Work out the finished part from the listing and answer in its coordinate system (mm). A direction names the side the tool comes from. Give positions to 0.01 mm unless a question says otherwise; leave off trailing zeros. Write each loop counter-clockwise with the first axis right and the second up, starting at its lowest first coordinate (ties: lowest second). Pieces come first, ordered by that corner, then holes. Notation, with made-up numbers: (-2.5, 41) -> (51.5, 41) arc R23 cw to (51.5, 60) -> close; hole circle Ø2 at (7, -38). An arc over 180 degrees is marked (long way). Use a Markdown table: item, result. Add a question column.
Q1. For a pull along Z with two mould halves and no side action, classify faces 1 (the face through (-6.2, -9.3, 0)), 2 (the face through (14, 0, 56)), 3 (the face through (-14, -8, 87)), 4 (the face through (13.57, -11.02, 38.6)) as pulls with the +Z half, pulls with the -Z half, needs draft (parallel to the pull), parting line crosses it, or undercut.
Q2. For faces 5 (the face through (18, -11, 25)), 6 (the face through (-12.27, -3.944, 27.444)), 7 (the face through (22.4, -6.41, 49.07)), 8 (the face through (-18, -7, 55)), determine the directions among +Z, -Z, +X, -X, +Y, -Y from which every point of the face is accessible in a straight line to the end or side of a thin tool.
Q3. Section B-B, the plane z = 56 is taken. Give the vertices of the cut face in (x, y) (3 decimals).
Q4. Each of these flat-tipped pins is pushed along its axis until it touches: pin 1 Ø6 at (x, z) = (-3.5, 17.5) entering from +Y; pin 2 Ø1.2 at (x, y) = (19, -11.5) entering from +Z; pin 3 Ø1.2 at (x, y) = (17.5, -11) entering from -Z; pin 4 Ø4.5 at (x, z) = (18, 31.5) entering from -Y. Where does it stop, or does it pass through?
Q5. Section C-C, the plane x = -14.5 is taken. Give the vertices of the cut face in (y, z) (3 decimals), plus the area to 3 significant figures.
Q6. Section D-D, the plane x = 0 is taken. Give the vertices of the cut face in (y, z), plus the area to 3 significant figures.
Q7. Section A-A, the plane z = 31.5 is taken. Give the vertices of the cut face in (x, y).
Q8. Consider line 1 (Z direction, x = 20.5, y = -9.25); line 2 (Z direction, x = -14.5, y = -2.5) (3 decimals); line 3 (Z direction, x = 18, y = -10.7). Determine where each line is inside the solid, lowest interval first.
from build123d import *

# Parameters (mm, degrees)
BOSS_EXTRUDE1_DEPTH  = 112
SKETCH2_R            = 3.025
CUT_EXTRUDE1_DEPTH   = 8
SKETCH3_W            = 11
SKETCH3_H            = 11
BOSS_EXTRUDE2_DEPTH  = 4
BOSS_EXTRUDE3_REACH  = 126.988
SKETCH8_W            = 10
SKETCH8_H            = 13
BOSS_EXTRUDE4_DEPTH  = 4
FILLET1_R            = 2
M4_CLEARANCE_HOLE1_D = 4.8
MIRROR1_START        = 12.831076745
MIRROR1_OUTLINE_W    = 4
MIRROR1_OUTLINE_H    = 13
MIRROR1_DEPTH        = 2.768923155
MIRROR1_START_2      = 20.4000001
MIRROR1_2_OUTLINE_W  = 4
MIRROR1_2_OUTLINE_H  = 13
MIRROR1_2_DEPTH      = 0.5999999
MIRROR1_START_3      = 74
MIRROR1_3_DEPTH      = 13
MIRROR1_4_OUTLINE_W  = 4.8000002
MIRROR1_4_OUTLINE_H  = 4
MIRROR1_4_DEPTH      = 4.0999999
MIRROR1_START_4      = 82.9000001
MIRROR1_5_OUTLINE_W  = 4.8000002
MIRROR1_5_OUTLINE_H  = 4
MIRROR1_5_DEPTH      = 4.0999999
MIRROR1_START_5      = 76
MIRROR1_6_OUTLINE_W  = 2
MIRROR1_6_OUTLINE_H  = 4
MIRROR1_6_DEPTH      = 9
MIRROR1_START_6      = -13
MIRROR1_7_DEPTH      = 4
CUT_EXTRUDE2_DEPTH   = 126.455171276
BOSS_EXTRUDE5_START  = -87
BOSS_EXTRUDE5_DEPTH  = 112
SKETCH15_W           = 10
SKETCH15_H           = 15
SKETCH15_R           = 3.025
BOSS_EXTRUDE6_DEPTH  = 13
SKETCH16_R           = 3.025
CUT_EXTRUDE3_DEPTH   = 8
FILLET2_R            = 2
FILLET3_R            = 1


with BuildPart() as part:
    # Sketch1 → Boss-Extrude1 (new body)
    with BuildSketch(Plane.XY):
        with BuildLine():
            ThreePointArc((0, -13), (-9.192388155, -9.192388155), (-13, 0))
            Line((-13, 0), (-18, 0))
            Line((-18, 0), (-18, -13))
            Line((-18, -13), (0, -13))
        make_face()
        with BuildLine():
            Line((-11, 0), (-13, 0))
            ThreePointArc((-13, 0), (-9.192388155, -9.192388155), (0, -13))
            ThreePointArc((0, -13), (9.192388155, -9.192388155), (13, 0))
            Line((13, 0), (11, 0))
            ThreePointArc((11, 0), (0, -11), (-11, 0))
        make_face()
    extrude(amount=BOSS_EXTRUDE1_DEPTH)

    # Sketch2 → Cut-Extrude1 (cut)
    with BuildSketch(Plane(origin=(0, 0, 0), x_dir=(1, 0, 0), z_dir=(0, 1, 0))):
        with Locations(Location((-14.5, -25.4, 0), (0, 0, 180))):
            Circle(SKETCH2_R)
        with Locations(Location((-14.5, -86.6, 0), (0, 0, 180))):
            Circle(SKETCH2_R)
    extrude(amount=-CUT_EXTRUDE1_DEPTH, mode=Mode.SUBTRACT)

    # Sketch3 → Boss-Extrude2 (add)
    with BuildSketch(Plane.XZ.offset(13)):
        with Locations((-12.5, 117.5)):
            Rectangle(SKETCH3_W, SKETCH3_H)
    extrude(amount=-BOSS_EXTRUDE2_DEPTH)

    # Sketch7 → Boss-Extrude3 (add, up to next)
    with BuildSketch(Plane.XZ.offset(13), mode=Mode.PRIVATE) as boss_extrude3_sk1:
        Polygon((0, 25), (13, 25), (13, 31.5), (13, 38), (0, 38), align=None)
    boss_extrude3_tool1 = extrude(boss_extrude3_sk1.sketch, amount=-BOSS_EXTRUDE3_REACH, mode=Mode.PRIVATE) - part.part
    add(boss_extrude3_tool1.solids().sort_by_distance((6.5, -13, 31.5))[0])

    # Sketch8 → Boss-Extrude4 (add)
    with BuildSketch(Plane.XZ.offset(13)):
        with Locations((18, 31.5)):
            Rectangle(SKETCH8_W, SKETCH8_H)
    extrude(amount=-BOSS_EXTRUDE4_DEPTH)

    # Fillet1
    fillet1_edges = [part.edges().sort_by_distance(p)[0] for p in [
        (-18, -11, 123),
        (-7, -11, 123),
        (23, -11, 38),
        (23, -11, 25),
    ]]
    fillet(fillet1_edges, radius=FILLET1_R)

    # M4 Clearance Hole1 (through all)
    with Locations(Plane(origin=(0, -9, 0), x_dir=(1, 0, 0), z_dir=(0, 1, 0))):
        with Locations((-12.5, -117.5), (18, -31.5)):
            Hole(M4_CLEARANCE_HOLE1_D / 2)



with BuildPart() as body_2:
    # Mirror1: read off the stored shape, not the designer's step
    # Mirror1 outline → Mirror1 (new body)
    with BuildSketch(Plane.YZ.offset(MIRROR1_START)):
        with Locations((-11, 80.5)):
            Rectangle(MIRROR1_OUTLINE_W, MIRROR1_OUTLINE_H)
    extrude(amount=MIRROR1_DEPTH)


with BuildPart() as body_3:
    # Mirror1 2 outline → Mirror1 2 (new body)
    with BuildSketch(Plane.YZ.offset(MIRROR1_START_2)):
        with Locations((-11, 80.5)):
            Rectangle(MIRROR1_2_OUTLINE_W, MIRROR1_2_OUTLINE_H)
    extrude(amount=MIRROR1_2_DEPTH)


with BuildPart() as part_1:
    add(part.part)

    add(body_2.part)  # Mirror1 3 merges body 2
    # Mirror1 3 outline → Mirror1 3 (add)
    with BuildSketch(Plane.XY.offset(MIRROR1_START_3)):
        with BuildLine():
            Line((15.5999999, -9), (13, -9))
            Line((13, -9), (13, 0))
            ThreePointArc((13, 0), (9.192388155, -9.192388155), (0, -13))
            Line((0, -13), (12.831076745, -13))
            Line((12.831076745, -13), (15.5999999, -13))
            Line((15.5999999, -13), (15.5999999, -9))
        make_face()
    extrude(amount=MIRROR1_3_DEPTH)


    add(body_3.part)  # Mirror1 4 merges body 3
    # Mirror1 4 outline → Mirror1 4 (add)
    with BuildSketch(Plane.XY.offset(MIRROR1_START_3)):
        with Locations((18, -11)):
            Rectangle(MIRROR1_4_OUTLINE_W, MIRROR1_4_OUTLINE_H)
    extrude(amount=MIRROR1_4_DEPTH)

    # Mirror1 5 outline → Mirror1 5 (add)
    with BuildSketch(Plane.XY.offset(MIRROR1_START_4)):
        with Locations((18, -11)):
            Rectangle(MIRROR1_5_OUTLINE_W, MIRROR1_5_OUTLINE_H)
    extrude(amount=MIRROR1_5_DEPTH)

    # Mirror1 6 outline → Mirror1 6 (add)
    with BuildSketch(Plane.XY.offset(MIRROR1_START_5)):
        with Locations((22, -11)):
            Rectangle(MIRROR1_6_OUTLINE_W, MIRROR1_6_OUTLINE_H)
    extrude(amount=MIRROR1_6_DEPTH)

    # Mirror1 7 outline → Mirror1 7 (add)
    with BuildSketch(Plane(origin=(0, 0, 0), x_dir=(1, 0, 0), z_dir=(0, 1, 0)).offset(MIRROR1_START_6)):
        with BuildLine():
            ThreePointArc((23, -76), (22.414213562, -74.585786438), (21, -74))
            Line((21, -74), (21, -76))
            Line((21, -76), (23, -76))
        make_face()
        with BuildLine():
            Line((21, -85), (21, -87))
            ThreePointArc((21, -87), (22.414213562, -86.414213562), (23, -85))
            Line((23, -85), (21, -85))
        make_face()
        with BuildLine():
            Line((20.4000001, -82.9000001), (20.4, -80.5))
            ThreePointArc((20.4, -80.5), (19.697056275, -82.197056275), (18, -82.9))
            Line((18, -82.9), (20.4000001, -82.9000001))
        make_face()
        with BuildLine():
            ThreePointArc((18, -78.1), (19.697056275, -78.802943725), (20.4, -80.5))
            Line((20.4, -80.5), (20.4000001, -78.0999999))
            Line((20.4000001, -78.0999999), (18, -78.1))
        make_face()
        with BuildLine():
            ThreePointArc((15.6, -80.5), (16.302943725, -78.802943725), (18, -78.1))
            Line((18, -78.1), (15.5999999, -78.0999999))
            Line((15.5999999, -78.0999999), (15.6, -80.5))
        make_face()
        with BuildLine():
            Line((15.5999999, -82.9000001), (18, -82.9))
            ThreePointArc((18, -82.9), (16.302943725, -82.197056275), (15.6, -80.5))
            Line((15.6, -80.5), (15.5999999, -82.9000001))
        make_face()
    extrude(amount=MIRROR1_7_DEPTH)

    # Sketch12 → Cut-Extrude2 (cut, through all)
    with BuildSketch(Plane(origin=(0, -9, 0), x_dir=(1, 0, 0), z_dir=(0, 1, 0))):
        with BuildLine():
            Line((-18, -112), (-18, -121))
            ThreePointArc((-18, -121), (-17.414213562, -122.414213562), (-16, -123))
            Line((-16, -123), (-9, -123))
            ThreePointArc((-9, -123), (-7.585786438, -122.414213562), (-7, -121))
            Line((-7, -121), (-7, -112))
            Line((-7, -112), (-18, -112))
        make_face()
    extrude(amount=-CUT_EXTRUDE2_DEPTH, mode=Mode.SUBTRACT)

    # Sketch13 → Boss-Extrude5 (add)
    with BuildSketch(Plane.XY.offset(87).offset(BOSS_EXTRUDE5_START)):
        with BuildLine():
            Line((13, -13), (13, -9))
            Line((13, -9), (13, 0))
            ThreePointArc((13, 0), (9.192388155, -9.192388155), (0, -13))
            Line((0, -13), (13, -13))
        make_face()
    extrude(amount=BOSS_EXTRUDE5_DEPTH)

    # Sketch15 → Boss-Extrude6 (add)
    # profile 1 of 2: a face of its own
    with BuildSketch(Plane.XZ.offset(13)):
        with Locations((18, 56)):
            Rectangle(SKETCH15_W, SKETCH15_H)
        with Locations((18, 56)):
            Circle(SKETCH15_R, mode=Mode.SUBTRACT)
    # profile 2 of 2: a face of its own
    with BuildSketch(Plane.XZ.offset(13)):
        with Locations((18, 56)):
            Circle(SKETCH15_R)
    extrude(amount=-BOSS_EXTRUDE6_DEPTH)

    # Sketch16 → Cut-Extrude3 (cut)
    with BuildSketch(Plane(origin=(0, 0, 0), x_dir=(1, 0, 0), z_dir=(0, 1, 0))):
        with Locations(Location((18, -56, 0), (0, 0, 270))):
            Circle(SKETCH16_R)
    extrude(amount=-CUT_EXTRUDE3_DEPTH, mode=Mode.SUBTRACT)

    # Fillet2
    fillet2_edges = [part_1.edges().sort_by_distance(p)[0] for p in [
        (13, -11, 25),
        (13, -11, 38),
        (13, -11, 74),
        (13, -11, 87),
        (23, -6.5, 63.5),
        (23, -6.5, 48.5),
        (13, -6.5, 48.5),
        (13, -6.5, 63.5),
    ]]
    fillet(fillet2_edges, radius=FILLET2_R)

    # Fillet3
    fillet3_edges = [part_1.edges().sort_by_distance(p)[0] for p in [
        (13, -9, 80.5),
        (13, -9, 31.5),
    ]]
    fillet(fillet3_edges, radius=FILLET3_R)


solid = part_1.part
Result set:
| question | item | result |
|---|---|---|
| 1 | face 1 | pulls with the -Z half |
| 1 | face 2 | needs draft |
| 1 | face 3 | undercut |
| 1 | face 4 | undercut |
| 2 | face 5 | -Z, +X, +Y, -Y |
| 2 | face 6 | +Y |
| 2 | face 7 | +X, +Y, -Y |
| 2 | face 8 | +Z, -Z, -X, +Y, -Y |
| 3 | outline | (-18, -13) -> (23, -13) -> (23, 0) -> (21.025, 0) -> (21.025, -8) -> (14.975, -8) -> (14.975, 0) -> (11, 0) arc R11 cw to (-11, 0) -> (-18, 0) -> close |
| 4 | pin 1 | stops at y = -8.87 |
| 4 | pin 2 | stops at z = 87 |
| 4 | pin 3 | stops at z = 25 |
| 4 | pin 4 | passes through |
| 5 | outline | (-13, 0) -> (0, 0) -> (0, 22.375) -> (-8, 22.375) -> (-8, 28.425) -> (0, 28.425) -> (0, 83.575) -> (-8, 83.575) -> (-8, 89.625) -> (0, 89.625) -> (0, 112) -> (-13, 112) -> close |
| 5 | area | 1,360 mm2 |
| 6 | outline | (-13, 0) -> (-11, 0) -> (-11, 112) -> (-13, 112) -> close |
| 6 | area | 224 mm2 |
| 7 | outline | (-18, -13) -> (15.6, -13) -> (15.6, -9) -> (14, -9) arc R1 cw to (13, -8) -> (13, 0) -> (11, 0) arc R11 cw to (-11, 0) -> (-18, 0) -> close; (20.4, -13) -> (23, -13) -> (23, -9) -> (20.4, -9) -> close |
| 8 | line 1 | z = 25 to 38, 48.5 to 63.5, 74 to 87 |
| 8 | line 2 | z = 0 to 22.375, 28.425 to 83.575, 89.625 to 112 |
| 8 | line 3 | z = 25 to 29.1, 33.9 to 38, 48.5 to 63.5, 74 to 78.1, 82.9 to 87 |
